The listing builds one solid part. Answer for the finished solid, in the listing's coordinates (mm). A direction names the side the tool comes from. Round coordinates to 2 decimals unless told otherwise and drop trailing zeros. Loops run counter-clockwise (first coordinate to the right, second up) from the corner with the lowest first, then second, coordinate; pieces in that order, holes last. Notation, with made-up numbers: M -11.5,-14 L 16.5,-14 A27 ccw 16.5,16 Z; hole C -26,-24.5 d8. An arc over 180 degrees is marked long. Answer as a JSON object with one key per item and string values.
```python
from build123d import *

# Parameters (mm, degrees)
F0_W     = 20
F0_H     = 8
F1_DEPTH = 1
F2_W     = 20
F2_H     = 8
F2_W_2   = 14
F2_H_2   = 0.5
F3_DEPTH = 10
F6_DEPTH = 14
F7_W     = 20
F7_H     = 8
F8_DEPTH = 2


with BuildPart() as f1:
    # F0 (on Top) → F1 (new body)
    with BuildSketch(Plane.XY):
        Rectangle(F0_W, F0_H)
    extrude(amount=F1_DEPTH)

    # F2 (on face) → F3 (join)
    with BuildSketch(Plane.XY.offset(1)):
        Rectangle(F2_W, F2_H)
        Rectangle(F2_W_2, F2_H_2, mode=Mode.SUBTRACT)
    extrude(amount=F3_DEPTH)

    # F5 (on face) → F6 (join, through all)
    with BuildSketch(Plane.YZ.offset(-7)):
        Polygon((0, 8.26), (0.25, 8.01), (0.25, 8.51), align=None)
        Polygon((-0.25, 8.01), (0, 8.26), (-0.25, 8.51), align=None)
        Polygon((-0.25, 8.51), (0, 8.26), (0.25, 8.51), (0.25, 11), (-0.25, 11), align=None)
        Polygon((0.25, 11), (0.25, 8.51), (2.74, 11), align=None)
        Polygon((-2.74, 11), (-0.25, 8.51), (-0.25, 11), align=None)
    extrude(amount=F6_DEPTH)

    # F7 (on face) → F8 (join)
    with BuildSketch(Plane.XY.offset(11)):
        Rectangle(F7_W, F7_H)
    extrude(amount=F8_DEPTH)


solid = f1.part
```
Item 1: Determine the mould class of faces 1 (the face through (0, -4, 6)), 2 (the face through (0, -0.25, 4)), 3 (the face through (0, 0, 0)) for opening direction Z: released by +Z, released by -Z, zero draft, split by the parting line, or undercut.
Values follow:
{"face 1": "zero draft", "face 2": "undercut", "face 3": "released by -Z"}
Item 2: Which of the six approach directions +Z, -Z, +X, -X, +Y, -Y give full straight-line access (tool end or side, diameter ignored) to faces 4 (the face through (0, 0, 13)), 5 (the face through (0, 0.25, 4))?
Values follow:
{"face 4": "+Z, +X, -X, +Y, -Y", "face 5": "none"}
Item 3: A straight line is drawn through the part: line 1 (Y direction, x = 2.5, z = 7). Find the intervals that lie inside material, in ascending order.
Values follow:
{"line 1": "-4 to -0.25, 0.25 to 4"}
Item 4: The part is cut by section A-A (z = 4.75). Give the vertices of the cut face in (x, y).
Values follow:
{"outline": "M -10,-4 L 10,-4 L 10,4 L -10,4 Z; hole M -7,-0.25 L 7,-0.25 L 7,0.25 L -7,0.25 Z"}
Item 5: The part is cut by section B-B (x = 4.5). Give the vertices of the cut face in (y, z), then the cut area to 3 significant figures.
Values follow:
{"outline": "M -4,0 L 4,0 L 4,13 L -4,13 Z; hole M -0.25,1 L 0.25,1 L 0.25,8.01 L 0,8.26 L -0.25,8.01 Z", "area": "100 mm^2"}
